```python
from build123d import *

# Parameters (mm, degrees)
F1_DEPTH       = 3.8862
F2_COUNT       = 8
F0_R           = 12.0523
F3_DEPTH       = 8.0518
F4_D           = 4.8006
F4_CBORE_D     = 6.731
F4_CBORE_DEPTH = 3.5306
F5_R           = 0.254
F6_DEPTH       = 3.8862


with BuildPart() as f1:
    # F0 (on Front) → F1 (new body)
    with BuildSketch(Plane.XZ):
        with BuildLine():
            Line((0.6985, 4.7623475976), (0.6985, 6.9467475976))
            Line((0.6985, 6.9467475976), (0.013371136, 6.9467475976))
            Line((0.013371136, 6.9467475976), (0, 6.9137418223))
            Line((0, 6.9137418223), (-0.013371136, 6.9467475976))
            Line((-0.013371136, 6.9467475976), (-0.6985, 6.9467475976))
            Line((-0.6985, 6.9467475976), (-0.6985, 4.7623475976))
            ThreePointArc((-0.6985, 4.7623475976), (0, 4.8133), (0.6985, 4.7623475976))
        make_face()
        with BuildLine():
            Line((0.6985, 6.9467475976), (2.1004446952, 10.4073564329))
            ThreePointArc((2.1004446952, 10.4073564329), (1.7808041825, 10.4667890159), (1.4594938078, 10.51640688))
            Line((1.4594938078, 10.51640688), (0.013371136, 6.9467475976))
            Line((0.013371136, 6.9467475976), (0.6985, 6.9467475976))
        make_face()
        with BuildLine():
            ThreePointArc((-1.4594938078, 10.51640688), (-1.7808041825, 10.4667890159), (-2.1004446952, 10.4073564329))
            Line((-2.1004446952, 10.4073564329), (-0.6985, 6.9467475976))
            Line((-0.6985, 6.9467475976), (-0.013371136, 6.9467475976))
            Line((-0.013371136, 6.9467475976), (-1.4594938078, 10.51640688))
        make_face()
    extrude(amount=F1_DEPTH)


with BuildPart() as f2_1:
    # F2: instance of F1
    add(f1.part.rotate(Axis((0, 0, 0), (0, -1, 0)), 1 * 360 / F2_COUNT))


with BuildPart() as f2_2:
    # F2: instance of F1
    add(f1.part.rotate(Axis((0, 0, 0), (0, -1, 0)), 2 * 360 / F2_COUNT))


with BuildPart() as f2_3:
    # F2: instance of F1
    add(f1.part.rotate(Axis((0, 0, 0), (0, -1, 0)), 3 * 360 / F2_COUNT))


with BuildPart() as f2_4:
    # F2: instance of F1
    add(f1.part.rotate(Axis((0, 0, 0), (0, -1, 0)), 4 * 360 / F2_COUNT))


with BuildPart() as f2_5:
    # F2: instance of F1
    add(f1.part.rotate(Axis((0, 0, 0), (0, -1, 0)), 5 * 360 / F2_COUNT))


with BuildPart() as f2_6:
    # F2: instance of F1
    add(f1.part.rotate(Axis((0, 0, 0), (0, -1, 0)), 6 * 360 / F2_COUNT))


with BuildPart() as f2_7:
    # F2: instance of F1
    add(f1.part.rotate(Axis((0, 0, 0), (0, -1, 0)), 7 * 360 / F2_COUNT))


with BuildPart() as f1_1:
    add(f1.part)

    add(f2_1.part)  # F3 merges F2_1

    add(f2_2.part)  # F3 merges F2_2

    add(f2_3.part)  # F3 merges F2_3

    add(f2_4.part)  # F3 merges F2_4

    add(f2_5.part)  # F3 merges F2_5

    add(f2_6.part)  # F3 merges F2_6

    add(f2_7.part)  # F3 merges F2_7
    # F0 (on Front) → F3 (join)
    with BuildSketch(Plane.XZ):
        Circle(F0_R)
        with BuildLine():
            ThreePointArc((2.1004446952, 10.4073564329), (8.2166227021, 6.7239904232), (10.6172, 0))
            ThreePointArc((10.6172, 0), (-6.7239904232, -8.2166227021), (-2.1004446952, 10.4073564329))
            ThreePointArc((-2.1004446952, 10.4073564329), (-1.7808041825, 10.4667890159), (-1.4594938078, 10.51640688))
            ThreePointArc((-1.4594938078, 10.51640688), (0, 10.6172), (1.4594938078, 10.51640688))
            ThreePointArc((1.4594938078, 10.51640688), (1.7808041825, 10.4667890159), (2.1004446952, 10.4073564329))
        make_face(mode=Mode.SUBTRACT)
        with BuildLine():
            ThreePointArc((4.8133, 0), (3.6421111282, 3.1468847167), (0.6985, 4.7623475976))
            Line((0.6985, 4.7623475976), (-0.6985, 4.7623475976))
            ThreePointArc((-0.6985, 4.7623475976), (-3.1468847167, -3.6421111282), (4.8133, 0))
        make_face()
    extrude(amount=F3_DEPTH)

    # F4 (through all)
    with Locations(Plane(origin=(0, 0, 0), x_dir=(1, 0, 0), z_dir=(0, 1, 0))):
        with Locations((0, 0)):
            CounterBoreHole(F4_D / 2, F4_CBORE_D / 2, F4_CBORE_DEPTH)

    # F5
    f5_edges = [f1_1.edges().sort_by_distance(p)[0] for p in [
        (-12.0523, -8.0518, 0),
        (-12.0523, 0, 0),
    ]]
    fillet(f5_edges, radius=F5_R)

    # F0 (on Front) → F6 (join, through all)
    with BuildSketch(Plane.XZ):
        with BuildLine():
            Line((-0.6985, 4.7623475976), (0.6985, 4.7623475976))
            ThreePointArc((0.6985, 4.7623475976), (0, 4.8133), (-0.6985, 4.7623475976))
        make_face()
    extrude(amount=F6_DEPTH)


solid = f1_1.part
```
The listing builds one solid part. Answer for the finished solid, in the listing's coordinates (mm). A direction names the side the tool comes from. Coordinates: 2 decimals unless noted, no trailing zeros. Write each loop counter-clockwise with the first axis right and the second up, starting at its lowest first coordinate (ties: lowest second). Pieces come first, ordered by that corner, then holes. Notation, with made-up numbers: M 70.5,8 L 129.5,8 A23 cw 129.5,40 Z; hole C 86,66.25 d5. An arc over 180 degrees is marked long. Use a Markdown table: item, result. Add a question column.
1. Section A-A (y = -7) is taken. Give the vertices of the cut face in (x, z), plus the area to 3 significant figures.
2. Given P1, Ø0.7, axis at x = -6.5, y = -2, coming from the +Z side; P2, Ø1.5, axis at x = -6.5, y = -6.5, coming from the -Z side; P3, Ø2, axis at x = 8.5, z = -9.5, coming from the -Y side; P4, Ø3.5, axis at x = 0, z = 7.5, coming from the -Y side, each flat-ended and moving along its own axis, determine where each tip first touches the part or whether it passes through.
3. Which of the six approach directions +Z, -Z, +X, -X, +Y, -Y give full straight-line access (tool end or side, diameter ignored) to faces 3 (the flat face through (7.149, -1.916, -5.156)), 4 (the flat face through (1.4, -3.531, 2.2)), 5 (the flat face through (6, -3.886, 5))?
4. Section B-B (y = -2) is taken. Count the separate pieces of the cut face and the enclosed holes in it, plus the area to 3 significant figures.
5. Straight lines are drawn through the part: line 1 along Z through (x, y) = (-2.75, -5.75); line 2 along Z through (x, y) = (-3.5, -7.25); line 3 along X through (y, z) = (-0.25, -3.5). For each, find the intervals that lie inside material, in ascending order. Write a range as [from, to].
6. For a pull along Z with two mould halves and no side action, classify faces 1 (the flat face through (-10, -8.052, 4)), 2 (the flat face through (-8.7, -1.92, -1.41)) as +Z half, -Z half, draft (parallel to the pull), parting line (faces both ways), or undercut.
Data:
| question | item | result |
|---|---|---|
| 1 | outline | C 0,0 d24.1; M -0.7,4.76 A4.81 ccw long 0.7,4.76 Z; hole C 0,0 d21.23; hole C 0,0 d4.8 |
| 1 | area | 157 mm2 |
| 2 | P1 | stops at z = 10.37 |
| 2 | P2 | stops at z = -10.59 |
| 2 | P3 | stops at y = -8.05 |
| 2 | P4 | stops at y = -3.89 |
| 3 | face 3 | +Y, -Y |
| 3 | face 4 | +Y |
| 3 | face 5 | -Y |
| 4 | separate pieces | 1 |
| 4 | enclosed holes | 17 |
| 4 | area | 202 mm2 |
| 5 | line 1 | z = [-11.73, -10.25], [-3.95, 3.95], [10.25, 11.73] |
| 5 | line 2 | z = [-11.53, -10.02], [-3.3, 3.3], [10.02, 11.53] |
| 5 | line 3 | x = [-11.53, -10.02], [-4.49, 4.49], [10.02, 11.53] |
| 6 | face 1 | draft |
| 6 | face 2 | undercut |
